Autodesk Inventor part; units mm, degrees
ref_plane "YZ Plane" through (0, 0, 0) normal (1, 0, 0) x (0, 1, 0)
ref_plane "XZ Plane" through (0, 0, 0) normal (0, 1, 0) x (-1, 0, 0)
ref_plane "XY Plane" through (0, 0, 0) normal (0, 0, 1) x (1, 0, 0)
sketch "スケッチ1" plane through (0, 0, 0) normal (0, 0, 1) x (1, 0, 0)
  line L0 (-30, -15) -> (30, -15)
  line L1 (30, -15) -> (30, 15)
  line L2 (30, 15) -> (-30, 15)
  line L3 (-30, 15) -> (-30, -15)
  line L4 (-30, -15) -> (30, 15) construction
  line L5 (30, -15) -> (-30, 15) construction
  line L6 (-27.7, 12.7) -> (27.7, 12.7)
  line L7 (27.7, 12.7) -> (27.7, -12.7)
  line L8 (27.7, -12.7) -> (-27.7, -12.7)
  line L9 (-27.7, -12.7) -> (-27.7, 12.7)
  point P0 (0, 0)
  dimension "d0" = 60
  dimension "d1" = 30
  dimension "d2" = 2.3
extrude "押し出し1" add sketch "スケッチ1" along normal mid plane 60
chamfer "面取り1" distance 30 angle 45 1 edges at (0, 15, -30)
sketch "スケッチ2" plane through (-30, -15, 30) normal (0, -1, 0) x (1, 0, 0)
  point P0 (30, -30)
  point P1 (30, -30)
hole "穴1" at (0, -15, 0) direction (0, 1, 0) diameter 15 depth 10 tip angle 118
properties part number "車軸受け2"
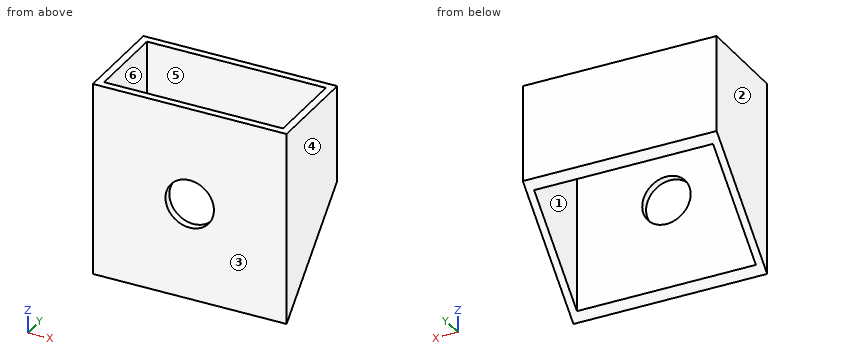
Geometry: final body of the model. Coordinates: model frame, mm. Face numbers are marked on the shaded views. A direction names the side the tool comes from. Round coordinates to 2 decimals unless told otherwise and drop trailing zeros. Loops run counter-clockwise (first coordinate to the right, second up) from the corner with the lowest first, then second, coordinate; pieces in that order, holes last. Notation, with made-up numbers: M 86.5,-21.75 L 98.5,-21.75 A18 ccw 98.5,-17.75 Z; hole C 39,-16.5 d2. An arc over 180 degrees is marked long. Put each result on its own line as item: value. Start each with the question number.
(1) Section query B-B (x = -22.5). Return loops of the section in (y, z), then the cut area to 3 significant figures.
(2) Contact query for flat-ended pins moving along their axis: pin 1 Ø12 at (x, z) = (12, -23) entering from +Y; pin 2 Ø6 at (x, y) = (-2.5, 9) entering from -Z. Output: stop coordinate, or through.
(3) Section query C-C (z = -24.5). Return loops of the section in (x, y), then the cut area to 3 significant figures.
(4) Section query D-D (z = -5). Return loops of the section in (x, y).
(5) Section query A-A (y = -5.5). Return loops of the section in (x, z), then the cut area to 3 significant figures.
(6) Material intervals for line 1 along Y through (x, z) = (5.5, 7); line 2 along X through (y, z) = (-13, 0); line 3 along X through (y, z) = (6, 17), sorted ascending. Write a range as [from, to].
(7) Draft query along Y for the marked faces 3, 4, 5 and 6. Return one class per face: +Y half, -Y half, draft (parallel to the pull), parting line (faces both ways), or undercut.
(8) Set-up query: the marked faces 1 and 2. Return all of +Z, -Z, +X, -X, +Y, -Y with unobstructed straight access to the full face (end or side cutting, diameter ignored); none if empty.
Findings below:
1. outline: M -15,-30 L -12.7,-27.7 L -12.7,30 L -15,30 Z; M 12.7,-2.3 L 15,0 L 15,30 L 12.7,30 Z
1. area: 207 mm2
2. pin 1: stops at y = -12.7
2. pin 2: passes through
3. outline: M -30,-15 L 30,-15 L 30,-9.5 L 27.7,-9.5 L 27.7,-12.7 L -27.7,-12.7 L -27.7,-9.5 L -30,-9.5 Z
3. area: 153 mm2
4. outline: M -30,-15 L -5.59,-15 L -5.59,-12.7 L -27.7,-12.7 L -27.7,10 L -30,10 Z; M 5.59,-15 L 30,-15 L 30,10 L 27.7,10 L 27.7,-12.7 L 5.59,-12.7 Z
5. outline: M -30,-20.5 L -27.7,-20.5 L -27.7,30 L -30,30 Z; M 27.7,-20.5 L 30,-20.5 L 30,30 L 27.7,30 Z
5. area: 232 mm2
6. line 1: y = [-15, -12.7], [12.7, 15]
6. line 2: x = [-30, -7.5], [7.5, 30]
6. line 3: x = [-30, -27.7], [27.7, 30]
7. face 3: -Y half
7. face 4: draft
7. face 5: undercut
7. face 6: undercut
8. face 1: +Z, -Z
8. face 2: +Z, -Z, -X, +Y, -Y
